```python
from build123d import *

# Parameters (mm, degrees)
F0_R     = 43.18
F1_DEPTH = 90.17
F0_R_2   = 59.055
F2_DEPTH = 6.35
F3_T     = -2.54
F4_R     = 43.18
F5_DEPTH = 3.81
F7_DEPTH = 3.81
F8_DEPTH = 2.54
F9_R     = 2.54
F10_R    = 1.524


with BuildPart() as f1:
    # F0 (on Top) → F1 (new body)
    with BuildSketch(Plane.XY):
        Circle(F0_R)
    extrude(amount=F1_DEPTH)

    # F0 (on Top) → F2 (join)
    with BuildSketch(Plane.XY):
        Circle(F0_R_2)
        Circle(F0_R, mode=Mode.SUBTRACT)
    extrude(amount=F2_DEPTH)

    # F3
    f3_openings = [f1.faces().sort_by_distance(p)[0] for p in [
        (0, 0, 90.17),
    ]]
    offset(amount=F3_T, openings=f3_openings, kind=Kind.INTERSECTION)

    # F4 (on face) → F5 (join)
    with BuildSketch(Plane.XY.offset(90.17)):
        Circle(F4_R)
    extrude(amount=F5_DEPTH)

    # F6 (on face) → F7 (cut, through all)
    with BuildSketch(Plane.XY.offset(93.98)):
        with BuildLine():
            ThreePointArc((-33.986308275, 0), (0, -33.986308275), (33.986308275, 0))
            ThreePointArc((33.986308275, 0), (0, 33.986308275), (-33.986308275, 0))
        make_face()
        with BuildLine():
            Line((33.986308275, 0), (36.9492512699, 0))
            ThreePointArc((36.9492512699, 0), (0, 36.9492512699), (-36.9492512699, 0))
            Line((-36.9492512699, 0), (-33.986308275, 0))
            ThreePointArc((-33.986308275, 0), (0, 33.986308275), (33.986308275, 0))
        make_face()
    extrude(amount=-F7_DEPTH, mode=Mode.SUBTRACT)

    # F6 (on face) → F8 (cut)
    with BuildSketch(Plane.XY.offset(93.98)):
        with BuildLine():
            ThreePointArc((-36.9492512699, 0), (0, -36.9492512699), (36.9492512699, 0))
            Line((36.9492512699, 0), (33.986308275, 0))
            ThreePointArc((33.986308275, 0), (0, -33.986308275), (-33.986308275, 0))
            Line((-33.986308275, 0), (-36.9492512699, 0))
        make_face()
    extrude(amount=-F8_DEPTH, mode=Mode.SUBTRACT)

    # F9
    f9_edges = [f1.edges().sort_by_distance(p)[0] for p in [
        (-59.055, 0, 6.35),
    ]]
    fillet(f9_edges, radius=F9_R)

    # F10
    f10_edges = [f1.edges().sort_by_distance(p)[0] for p in [
        (-43.18, 0, 93.98),
    ]]
    fillet(f10_edges, radius=F10_R)


solid = f1.part
```
Geometry: final body of the model. Coordinates: model frame, mm. A direction names the side the tool comes from. Coordinates: 2 decimals unless noted, no trailing zeros. Order: outer loops, then holes, each group sorted by start corner. A loop starts at its lowest first (then second) coordinate and runs counter-clockwise, first axis right, second up.
Item 1: Material intervals for line 1 along Y through (x, z) = (0, 3.45) (3 decimals); line 2 along Z through (x, y) = (38.5, -20); line 3 along Y through (x, z) = (0, 27.5), sorted ascending.
Answer:
line 1: y = -59.055 to -56.515, 56.515 to 59.055
line 2: z = 0 to 2.54, 3.81 to 6.35
line 3: y = -43.18 to -40.64, 40.64 to 43.18
Item 2: Section query A-A (x = 0). Output: boundary loops of the cut face in (y, z) (3 decimals).
Answer:
outline: (-59.055, 0) - (59.055, 0) - (59.055, 3.81) arc R2.54 ccw to (56.515, 6.35) - (43.18, 6.35) - (43.18, 92.456) arc R1.524 ccw to (41.656, 93.98) - (36.949, 93.98) - (36.949, 90.17) - (40.64, 90.17) - (40.64, 3.81) - (56.515, 3.81) - (56.515, 2.54) - (-56.515, 2.54) - (-56.515, 3.81) - (-40.64, 3.81) - (-40.64, 90.17) - (-33.986, 90.17) - (-33.986, 91.44) - (-36.949, 91.44) - (-36.949, 93.98) - (-41.656, 93.98) arc R1.524 ccw to (-43.18, 92.456) - (-43.18, 6.35) - (-56.515, 6.35) arc R2.54 ccw to (-59.055, 3.81) - close
Item 3: Contact query for flat-ended pins moving along their axis: P1, Ø3, axis at y = 19.5, z = 77, coming from the -X side; P2, Ø18.5, axis at x = 15, y = -16, coming from the +Z side; P3, Ø10, axis at y = 15, z = 57.5, coming from the -X side; P4, Ø2, axis at x = -41.5, y = -0.5, coming from the -Z side. Output: stop coordinate, or through.
Answer:
P1: stops at x = -39.25
P2: stops at z = 2.54
P3: stops at x = -42.01
P4: stops at z = 0
Item 4: Section query B-B (z = 64). Output: boundary loops of the cut face in (x, y), then the cut area to 3 significant figures.
Answer:
outline: circle Ø86.36 at (0, 0); hole circle Ø81.28 at (0, 0)
area: 669 mm2
Item 5: Access query for faces 1 (the face through (-17.05, 32.78, 92.53)), 2 (the face through (-9, -33, 90.17)). Directions: +Z, -Z, +X, -X, +Y, -Y. A direction counts if a zero-diameter tool reaches every point of the face in a straight line with its end or side. Return the directions, or none.
Answer:
face 1: +Z
face 2: none
Item 6: Draft query along Z for faces 3 (the face through (54.55, -22.62, 1.88)), 4 (the face through (-1, 1, 0)), 5 (the face through (37, -24, 3.81)), 6 (the face through (-16, -34, 93.98)). Return one class per face: released by +Z, released by -Z, zero draft, split by the parting line, or undercut.
Answer:
face 3: zero draft
face 4: released by -Z
face 5: undercut
face 6: released by +Z
